from build123d import *

# Parameters (mm, degrees)
SKETCH1_W           = 40
SKETCH1_H           = 40
BOSS_EXTRUDE2_DEPTH = 1.5
SKETCH2_W           = 40
SKETCH2_H           = 40
SKETCH2_W_2         = 37
SKETCH2_H_2         = 37
BOSS_EXTRUDE3_DEPTH = 37
SKETCH3_W           = 40
SKETCH3_H           = 40
BOSS_EXTRUDE4_DEPTH = 1.5
SKETCH4_R           = 7.5
CUT_EXTRUDE1_DEPTH  = 70.282032303
SKETCH5_R           = 7.5
CUT_EXTRUDE2_DEPTH  = 69.426968368
SKETCH6_R           = 7.5
CUT_EXTRUDE3_DEPTH  = 69.426968368


with BuildPart() as part:
    # Sketch1 → Boss-Extrude2 (new body)
    with BuildSketch(Plane(origin=(0, 0, 0), x_dir=(1, 0, 0), z_dir=(0, 1, 0))):
        with Locations((20, 20)):
            Rectangle(SKETCH1_W, SKETCH1_H)
    extrude(amount=-BOSS_EXTRUDE2_DEPTH)

    # Sketch2 → Boss-Extrude3 (add)
    with BuildSketch(Plane(origin=(0, 0, 0), x_dir=(1, 0, 0), z_dir=(0, 1, 0))):
        with Locations((20, 20)):
            Rectangle(SKETCH2_W, SKETCH2_H)
        with Locations((20, 20)):
            Rectangle(SKETCH2_W_2, SKETCH2_H_2, mode=Mode.SUBTRACT)
    extrude(amount=BOSS_EXTRUDE3_DEPTH)

    # Sketch3 → Boss-Extrude4 (add)
    with BuildSketch(Plane(origin=(0, 37, 0), x_dir=(1, 0, 0), z_dir=(0, 1, 0))):
        with Locations((20, 20)):
            Rectangle(SKETCH3_W, SKETCH3_H)
    extrude(amount=BOSS_EXTRUDE4_DEPTH)

    # Sketch4 → Cut-Extrude1 (cut, through all)
    with BuildSketch(Plane(origin=(0, 38.5, 0), x_dir=(1, 0, 0), z_dir=(0, 1, 0))):
        with Locations(Location((20, 20, 0), (0, 0, 270))):
            Circle(SKETCH4_R)
    extrude(amount=-CUT_EXTRUDE1_DEPTH, mode=Mode.SUBTRACT)

    # Sketch5 → Cut-Extrude2 (cut, through all)
    with BuildSketch(Plane(origin=(40, 0, 0), x_dir=(0, 0, -1), z_dir=(1, 0, 0))):
        with Locations((20, 18.5)):
            Circle(SKETCH5_R)
    extrude(amount=-CUT_EXTRUDE2_DEPTH, mode=Mode.SUBTRACT)

    # Sketch6 → Cut-Extrude3 (cut, through all)
    with BuildSketch(Plane.XY):
        with Locations((20, 18.5)):
            Circle(SKETCH6_R)
    extrude(amount=-CUT_EXTRUDE3_DEPTH, mode=Mode.SUBTRACT)


solid = part.part
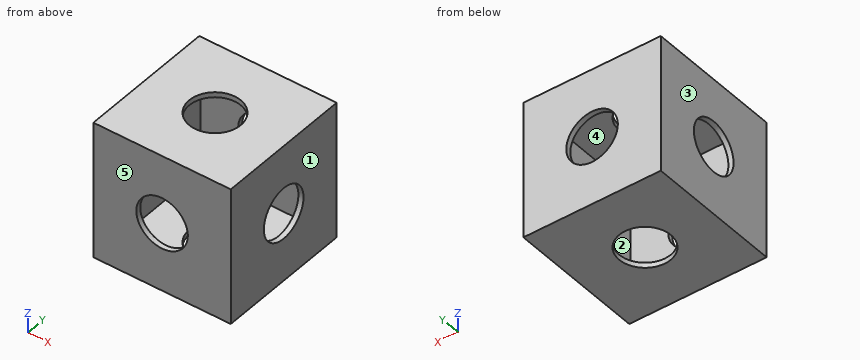
Verification items for the finished model (mm, model axes). Face numbers are marked on the shaded views. A direction names the side the tool comes from. Give positions to 0.01 mm unless a question says otherwise; leave off trailing zeros. Order: outer loops, then holes, each group sorted by start corner. A loop starts at its lowest first (then second) coordinate and runs counter-clockwise, first axis right, second up. Notation, with made-up numbers: (-6.75, 52.25) -> (-2.75, 52.25) arc R25 cw to (-2.75, 79.25) -> close; hole circle Ø3 at (71.25, 42.5). An arc over 180 degrees is marked (long way). Answer as CSV lines item,"result".
Q1. Depth check by flat-ended pin: pin 1 (9 mm diameter, centred on y = 18.5, z = -20, fed in from -X). Enter the tip coordinate at first touch or a pass-through.
Solutions:
pin 1,"passes through"
Q2. Scan lines: probe 1 along Z at (x, y) = (35, 27); probe 2 along X at (y, z) = (2.5, -11.5); probe 3 along Y at (x, z) = (29, -18). Record each from-to range of solid material in increasing order.
Solutions:
probe 1,"z = -40 to -38.5, -1.5 to 0"
probe 2,"x = 0 to 1.5, 38.5 to 40"
probe 3,"y = -1.5 to 0, 37 to 38.5"
Q3. Release check for a two-part mould opening along X. For the marked faces 3, 4 and 5 record: +X half, -X half, draft (parallel to the pull), parting line (faces both ways), or undercut.
Solutions:
face 3,"-X half"
face 4,"undercut"
face 5,"draft"
Q4. Access from +Z, -Z, +X, -X, +Y, -Y to the whole of each face (thin tool, end or side, straight path). Record for the marked faces 1 and 2.
Solutions:
face 1,"+Z, -Z, +X, +Y, -Y"
face 2,"none"
Q5. Sectioned sample at B-B on z = -14. Record the cut outline in (x, y).
Solutions:
outline,"(0, -1.5) -> (15.5, -1.5) -> (15.5, 0) -> (1.5, 0) -> (1.5, 14) -> (0, 14) -> close; (0, 23) -> (1.5, 23) -> (1.5, 37) -> (15.5, 37) -> (15.5, 38.5) -> (0, 38.5) -> close; (24.5, -1.5) -> (40, -1.5) -> (40, 14) -> (38.5, 14) -> (38.5, 0) -> (24.5, 0) -> close; (24.5, 37) -> (38.5, 37) -> (38.5, 23) -> (40, 23) -> (40, 38.5) -> (24.5, 38.5) -> close"
Q6. Sectioned sample at A-A on x = 20. Record the cut outline in (y, z), plus the area to 3 significant figures.
Solutions:
outline,"(-1.5, -40) -> (11, -40) -> (11, -38.5) -> (0, -38.5) -> (0, -27.5) -> (-1.5, -27.5) -> close; (-1.5, -12.5) -> (0, -12.5) -> (0, -1.5) -> (11, -1.5) -> (11, 0) -> (-1.5, 0) -> close; (26, -40) -> (38.5, -40) -> (38.5, -27.5) -> (37, -27.5) -> (37, -38.5) -> (26, -38.5) -> close; (26, -1.5) -> (37, -1.5) -> (37, -12.5) -> (38.5, -12.5) -> (38.5, 0) -> (26, 0) -> close"
area,"141 mm²"
Q7. Sectioned sample at C-C on x = 29.5. Record the cut outline in (y, z).
Solutions:
outline,"(-1.5, -40) -> (38.5, -40) -> (38.5, 0) -> (-1.5, 0) -> close; hole (0, -38.5) -> (37, -38.5) -> (37, -1.5) -> (0, -1.5) -> close"
Q8. Sectioned sample at D-D on z = -3.5. Record the cut outline in (x, y), plus the area to 3 significant figures.
Solutions:
outline,"(0, -1.5) -> (40, -1.5) -> (40, 38.5) -> (0, 38.5) -> close; hole (1.5, 0) -> (38.5, 0) -> (38.5, 37) -> (1.5, 37) -> close"
area,"231 mm²"
